```python
from build123d import *

# Parameters (mm, degrees)
SKETCH1_W           = 600
SKETCH1_H           = 801
BOSS_EXTRUDE1_DEPTH = 30.8


with BuildPart() as part:
    # Sketch1 → Boss-Extrude1 (new body)
    with BuildSketch(Plane(origin=(0, 0, 1970), x_dir=(-1, 0, 0), z_dir=(0, 0, -1))):
        with Locations((0, 24.5)):
            Rectangle(SKETCH1_W, SKETCH1_H)
        with BuildLine():
            Line((256.75, 393), (256.75, 307))
            ThreePointArc((256.75, 307), (253.25, 303.5), (256.75, 300))
            Line((256.75, 300), (280.55, 300))
            ThreePointArc((280.55, 300), (284.05, 303.5), (280.55, 307))
            Line((280.55, 307), (280.55, 393))
            ThreePointArc((280.55, 393), (284.05, 396.5), (280.55, 400))
            Line((280.55, 400), (256.75, 400))
            ThreePointArc((256.75, 400), (253.25, 396.5), (256.75, 393))
        make_face(mode=Mode.SUBTRACT)
        with BuildLine():
            Line((-256.75, 300), (-280.55, 300))
            ThreePointArc((-280.55, 300), (-284.05, 303.5), (-280.55, 307))
            Line((-280.55, 307), (-280.55, 393))
            ThreePointArc((-280.55, 393), (-284.05, 396.5), (-280.55, 400))
            Line((-280.55, 400), (-256.75, 400))
            ThreePointArc((-256.75, 400), (-253.25, 396.5), (-256.75, 393))
            Line((-256.75, 393), (-256.75, 307))
            ThreePointArc((-256.75, 307), (-253.25, 303.5), (-256.75, 300))
        make_face(mode=Mode.SUBTRACT)
        with BuildLine():
            Line((-256.75, -344), (-256.75, -258))
            ThreePointArc((-256.75, -258), (-253.25, -254.5), (-256.75, -251))
            Line((-256.75, -251), (-280.55, -251))
            ThreePointArc((-280.55, -251), (-284.05, -254.5), (-280.55, -258))
            Line((-280.55, -258), (-280.55, -344))
            ThreePointArc((-280.55, -344), (-284.05, -347.5), (-280.55, -351))
            Line((-280.55, -351), (-256.75, -351))
            ThreePointArc((-256.75, -351), (-253.25, -347.5), (-256.75, -344))
        make_face(mode=Mode.SUBTRACT)
        with BuildLine():
            Line((256.75, -251), (280.55, -251))
            ThreePointArc((280.55, -251), (284.05, -254.5), (280.55, -258))
            Line((280.55, -258), (280.55, -344))
            ThreePointArc((280.55, -344), (284.05, -347.5), (280.55, -351))
            Line((280.55, -351), (256.75, -351))
            ThreePointArc((256.75, -351), (253.25, -347.5), (256.75, -344))
            Line((256.75, -344), (256.75, -258))
            ThreePointArc((256.75, -258), (253.25, -254.5), (256.75, -251))
        make_face(mode=Mode.SUBTRACT)
    extrude(amount=-BOSS_EXTRUDE1_DEPTH)


solid = part.part
```
Input: part model. Units: mm. Frame: model coordinates. A direction names the side the tool comes from. Give positions to 0.01 mm unless a question says otherwise; leave off trailing zeros.
1. Reachability of faces 5 (the flat face through (4, 30, 2000.8)), 6 (the flat face through (-269, -351, 1985)) from +Z, -Z, +X, -X, +Y, -Y: full face, straight path, thin tool, end or side. Return the list, or none.
Derived:
face 5: +Z, +X, -X, +Y, -Y
face 6: +Z, -Z
2. Section A-A on z = 1990.5. Give the number of separate pieces and of enclosed holes in the cut face, and give its area (3 significant figures).
Derived:
separate pieces: 1
enclosed holes: 4
area: 471,000 mm2
3. Mould query, pull axis X, two halves, no side actions, for faces 1 (the flat face through (300, 19, 1985)), 2 (the flat face through (4, -376, 1985)), 3 (the flat face through (268, -251, 1985)), 4 (the flat face through (-280.55, -300, 1985)). Classes: released by +X, released by -X, zero draft, split by the parting line, or undercut.
Derived:
face 1: released by +X
face 2: zero draft
face 3: undercut
face 4: undercut
4. Material intervals for L1, parallel to X at y = -260, z = 1999; L2, parallel to Y at x = 255, z = 1997.5, sorted ascending.
Derived:
L1: x = -300 to -280.55, -256.75 to 256.75, 280.55 to 300
L2: y = -376 to -350.53, -344.47 to -257.53, -251.47 to 300.47, 306.53 to 393.47, 399.53 to 425
